Source: CAD feature listing. Evaluate the final solid. Frame: model axes, mm. Face numbers are marked on the shaded views. A direction names the side the tool comes from. Give positions to 0.01 mm unless a question says otherwise; leave off trailing zeros. Loops run counter-clockwise (first coordinate to the right, second up) from the corner with the lowest first, then second, coordinate; pieces in that order, holes last.
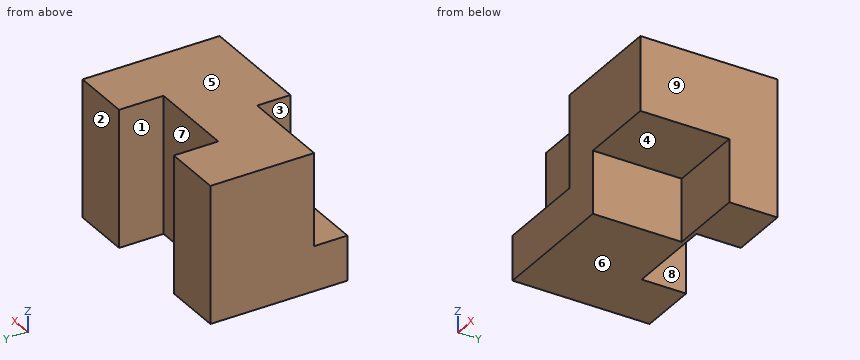
```python
from build123d import *

# Parameters (mm, degrees)
F1_DEPTH = 37.0078
F2_W     = 24.9682
F2_H     = 8.9916
F3_DEPTH = 24.9428
F4_W     = 24.003
F4_H     = 16.9418
F5_DEPTH = 20.8534


with BuildPart() as f1:
    # F0 (on Top) → F1 (new body)
    with BuildSketch(Plane.XY):
        Polygon((0, 37.0078), (0, 0), (56.007, 0), (56.007, 37.0078), (40.005, 37.0078), (40.005, 25.019), (16.002, 25.019), (16.002, 37.0078), align=None)
    extrude(amount=F1_DEPTH)

    # F2 (on face) → F3 (cut)
    with BuildSketch(Plane.XY.offset(37.0078)):
        with Locations((12.4841, 4.4958)):
            Rectangle(F2_W, F2_H)
    extrude(amount=-F3_DEPTH, mode=Mode.SUBTRACT)

    # F4 (on face) → F5 (cut)
    with BuildSketch(Plane.YZ.offset(56.007)):
        with Locations((12.0015, 8.4709)):
            Rectangle(F4_W, F4_H)
    extrude(amount=-F5_DEPTH, mode=Mode.SUBTRACT)


solid = f1.part
```
(1) Ray query, line 1 along X through (y, z) = (34, 33) (3 decimals); line 2 along Y through (x, z) = (35.5, 17); line 3 along Y through (x, z) = (17, 18). Return the intervals inside material, ascending.
A:
line 1: x = 0 to 16.002, 40.005 to 56.007
line 2: y = 0 to 25.02
line 3: y = 8.99 to 25.02
(2) Mould query, pull axis X, two halves, no side actions, for the marked faces 6, 7, 8 and 9. Classes: pulls with the +X half, pulls with the -X half, needs draft (parallel to the pull), parting line crosses it, or undercut.
A:
face 6: needs draft
face 7: undercut
face 8: undercut
face 9: pulls with the +X half
(3) First-contact query: pin 1 (5 mm diameter, centred on x = 47, y = 31.5, fed in from -Z); pin 2 (8 mm diameter, centred on x = 20.5, z = 7, fed in from +Y); pin 3 (13.5 mm diameter, centred on y = 7, z = 6, fed in from +X); pin 4 (10 mm diameter, centred on x = 50, z = 11.5, fed in from -Y). Flat tips, straight axial feed; report the tip coordinate or a pass-through.
A:
pin 1: stops at z = 0
pin 2: stops at y = 25.02
pin 3: stops at x = 35.15
pin 4: stops at y = 24
(4) Reachability of the marked faces 1, 2, 3, 4 and 5 from +Z, -Z, +X, -X, +Y, -Y: full face, straight path, thin tool, end or side. Return the list, or none.
A:
face 1: +Z, -Z, +Y
face 2: +Z, -Z, +X, -X, +Y
face 3: +Z, -X, -Y
face 4: -Z, +X, -Y
face 5: +Z, +X, -X, +Y, -Y
(5) Section A-A, the plane y = 29.5. Return the cut outline in (x, z) (3 decimals).
A:
outline: (0, 0) - (16.002, 0) - (16.002, 37.008) - (0, 37.008) - close; (40.005, 0) - (56.007, 0) - (56.007, 37.008) - (40.005, 37.008) - close
(6) Section B-B, the plane z = 34. Return the cut outline in (x, y) (3 decimals), then the cut area to 3 significant figures.
A:
outline: (0, 8.992) - (24.968, 8.992) - (24.968, 0) - (56.007, 0) - (56.007, 37.008) - (40.005, 37.008) - (40.005, 25.019) - (16.002, 25.019) - (16.002, 37.008) - (0, 37.008) - close
area: 1,560 mm2
(7) Section D-D, the plane y = 4. Return the cut outline in (x, z) (3 decimals).
A:
outline: (0, 0) - (35.154, 0) - (35.154, 16.942) - (56.007, 16.942) - (56.007, 37.008) - (24.968, 37.008) - (24.968, 12.065) - (0, 12.065) - close
(8) Section C-C, the plane x = 4. Return the cut outline in (y, z) (3 decimals).
A:
outline: (0, 0) - (37.008, 0) - (37.008, 37.008) - (8.992, 37.008) - (8.992, 12.065) - (0, 12.065) - close
